Here's how the part is built. I have some questions about the finished solid (model axes, mm). Face numbers are marked on the shaded views. A direction names the side the tool comes from. Give positions to 0.01 mm unless a question says otherwise; leave off trailing zeros. Write each loop counter-clockwise with the first axis right and the second up, starting at its lowest first coordinate (ties: lowest second). Pieces come first, ordered by that corner, then holes. Notation, with made-up numbers: (87.25, 45) -> (113.25, 45) arc R22 cw to (113.25, 55) -> close; hole circle Ø9 at (88, 61). An arc over 180 degrees is marked (long way). Use one line per item in the form item = value.
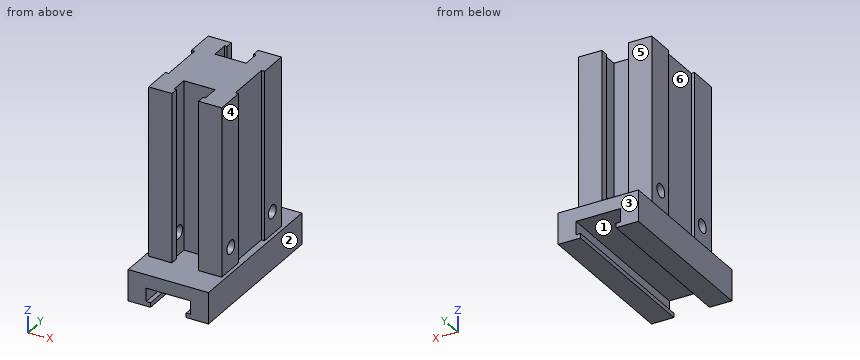
Autodesk Inventor part; units mm, degrees
ref_plane "XY Plane" through (0, 0, 0) normal (0, 0, 1) x (1, 0, 0)
sketch "Sketch1" plane through (0, 0, 0) normal (0, 0, 1) x (1, 0, 0)
  line L0 (8.2, -11.5) -> (-8.2, -11.5)
  line L1 (-8.2, -11.5) -> (-8.2, 11.5)
  line L2 (-8.2, 11.5) -> (8.2, 11.5)
  line L3 (8.2, 11.5) -> (8.2, -11.5)
  line L4 (8.2, -11.5) -> (-8.2, 11.5) construction
  line L5 (-8.2, -11.5) -> (8.2, 11.5) construction
  line L6 (8.2, -5) -> (-8.2, -5)
  line L7 (-8.2, -5) -> (-8.2, 5)
  line L8 (-8.2, 5) -> (8.2, 5)
  line L9 (8.2, 5) -> (8.2, -5)
  line L10 (8.2, -5) -> (-8.2, 5) construction
  line L11 (-8.2, -5) -> (8.2, 5) construction
  line L12 (7.5, -5) -> (-7.5, -5)
  line L13 (-7.5, -5) -> (-7.5, 5)
  line L14 (-7.5, 5) -> (7.5, 5)
  line L15 (7.5, 5) -> (7.5, -5)
  line L16 (7.5, -5) -> (-7.5, 5) construction
  line L17 (-7.5, -5) -> (7.5, 5) construction
  line L18 (3, -11.5) -> (-3, -11.5)
  line L19 (-3, -11.5) -> (-3, 11.5)
  line L20 (-3, 11.5) -> (3, 11.5)
  line L21 (3, 11.5) -> (3, -11.5)
  line L22 (3, -11.5) -> (-3, 11.5) construction
  line L23 (-3, -11.5) -> (3, 11.5) construction
  line L24 (3.5, -9.75) -> (-3.5, -9.75)
  line L25 (-3.5, -9.75) -> (-3.5, 9.75)
  line L26 (-3.5, 9.75) -> (3.5, 9.75)
  line L27 (3.5, 9.75) -> (3.5, -9.75)
  line L28 (3.5, -9.75) -> (-3.5, 9.75) construction
  line L29 (-3.5, -9.75) -> (3.5, 9.75) construction
  line L30 (3.5, -6) -> (-3.5, -6)
  line L31 (-3.5, -6) -> (-3.5, 6)
  line L32 (-3.5, 6) -> (3.5, 6)
  line L33 (3.5, 6) -> (3.5, -6)
  line L34 (3.5, -6) -> (-3.5, 6) construction
  line L35 (-3.5, -6) -> (3.5, 6) construction
  point P0 (0, 0)
  point P1 (-3, -9.75)
  point P2 (3, -9.75)
  point P3 (3, 9.75)
  point P4 (-3, 9.75)
  dimension "d0" = 23
  dimension "d1" = 16.4
  dimension "d2" = 10
  dimension "d3" = 15
  dimension "d4" = 6
  dimension "d5" = 19.5
  dimension "d6" = 7
  dimension "d7" = 12
extrude "Extrusion1" add sketch "Sketch1" along normal blind 37.8 contours L0 L21 L24 L27 L6 L3 | L0 L1 L6 L25 L24 L19 | L8 L27 L26 L21 L2 L3 | L6 L27 L8 L15 | L30 L19 L6 L21 | L21 L6 L27 L30 | L6 L21 L8 L27 | L30 L25 L6 L19 | L6 L19 L8 L21 | L8 L21 L32 L27 | L1 L2 L19 L26 L25 L8 | L13 L8 L25 L6 | L6 L25 L8 L19 | L8 L19 L32 L21 | L8 L25 L32 L19
sketch "Sketch2" plane through (0, 0, 0) normal (1, 0, 0) x (0, 1, 0)
  circle A0 centre (-8, 5) radius 1.5
  circle A1 centre (8, 5) radius 1.5
  line L0 (-6, 0) -> (-6, 37.8)
  line L1 (6, 10) -> (-6, 10)
  line L2 (-6, 10) -> (-6, 0)
  line L3 (-6, 0) -> (6, 0)
  line L4 (6, 0) -> (6, 10)
  line L5 (6, 10) -> (-6, 0) construction
  line L6 (-6, 10) -> (6, 0) construction
  point P0 (0, 0)
  point P1 (0, 5)
  point P2 (-6, 10)
  dimension "d10" = 3
  dimension "d11" = 3
  dimension "d12" = 16
  dimension "d13" = 8
  dimension "d14" = 5
  dimension "d17" = 10
extrude "Extrusion2" cut sketch "Sketch2" along normal through all both and the other way through all contours A0 | A1
sketch "Sketch3" plane through (0, 0, 0) normal (0, 0, -1) x (-1, 0, 0)
  line L0 (5, 18) -> (-5, 18)
  line L1 (-5, 18) -> (-5, -18)
  line L2 (-5, -18) -> (5, -18)
  line L3 (5, -18) -> (5, 18)
  line L4 (5, 18) -> (-5, -18) construction
  line L5 (-5, 18) -> (5, -18) construction
  line L6 (9, 18) -> (-9, 18)
  line L7 (-9, 18) -> (-9, -18)
  line L8 (-9, -18) -> (9, -18)
  line L9 (9, -18) -> (9, 18)
  line L10 (9, 18) -> (-9, -18) construction
  line L11 (-9, 18) -> (9, -18) construction
  line L12 (4, 18) -> (-4, 18)
  line L13 (-4, 18) -> (-4, -18)
  line L14 (-4, -18) -> (4, -18)
  line L15 (4, -18) -> (4, 18)
  line L16 (4, 18) -> (-4, -18) construction
  line L17 (-4, 18) -> (4, -18) construction
  point P0 (0, 0)
  point P1 (0, 18)
  point P2 (-5, 18)
  dimension "d20" = 10
  dimension "d21" = 18
  dimension "d22" = 36
  dimension "d23" = 36
  dimension "d24" = 8
extrude "Extrusion4" add sketch "Sketch3" along normal blind 7 contours L3 L2 L15 L0 | L6 L9 L8 L3 | L13 L2 L1 L0 | L1 L8 L7 L6
extrude "Extrusion5" cut sketch "Sketch3" along normal blind 6 contours L3 L2 L15 L0 | L13 L2 L1 L0
extrude "Extrusion6" add sketch "Sketch3" along normal blind 3 contours L3 L2 L15 L0 | L15 L2 L13 L0 | L13 L2 L1 L0
properties part number "Cylinder" material "Aluminum 6061"
Q1. I want a section at C-C, the plane x = -1.75. Write out the boundary of the cut face in (y, z), and give its area (3 significant figures).
Result set:
outline = (-18, -3) -> (18, -3) -> (18, 0) -> (6, 0) -> (6, 37.8) -> (-6, 37.8) -> (-6, 0) -> (-18, 0) -> close
area = 562 mm2
Q2. Will these pins go through, and if not, where does the flat tip stop? pin 1 Ø4 at (x, z) = (-5.5, 11) entering from +Y; pin 2 Ø4 at (y, z) = (8.5, 11) entering from -X; pin 3 Ø8 at (y, z) = (14, 28) entering from +X; pin 4 Ø2.5 at (y, z) = (8, 5) entering from +X.
Result set:
pin_1 = 11.5
pin_2 = -8.2
pin_3 = 8.2
pin_4 = through
Q3. Which directions (+Z, -Z, +X, -X, +Y, -Y) give clear straight access to the entire face, cutting with the end or side of a thin tool? Please do the marked faces 4, 5 and 6.
Result set:
face_4 = +Z, +X, +Y, -Y
face_5 = +Z, +X, -X, +Y
face_6 = +Z, -X
Q4. If we mould it in two halves opening along X, with no side actions, what happens to the marked faces 1, 2 and 3? For each: +X half, -X half, draft (parallel to the pull), parting line (faces both ways), or undercut.
Result set:
face_1 = undercut
face_2 = +X half
face_3 = draft
Q5. I want a section at D-D, the plane z = 12.5. Write out the boundary of the cut face in (x, y), and give its area (3 significant figures).
Result set:
outline = (-8.2, -11.5) -> (-3, -11.5) -> (-3, -9.75) -> (-3.5, -9.75) -> (-3.5, -6) -> (3.5, -6) -> (3.5, -9.75) -> (3, -9.75) -> (3, -11.5) -> (8.2, -11.5) -> (8.2, -5) -> (7.5, -5) -> (7.5, 5) -> (8.2, 5) -> (8.2, 11.5) -> (3, 11.5) -> (3, 9.75) -> (3.5, 9.75) -> (3.5, 6) -> (-3.5, 6) -> (-3.5, 9.75) -> (-3, 9.75) -> (-3, 11.5) -> (-8.2, 11.5) -> (-8.2, 5) -> (-7.5, 5) -> (-7.5, -5) -> (-8.2, -5) -> close
area = 290 mm2
Q6. I want a section at A-A, the plane x = 5.5. Write out the boundary of the cut face in (y, z), and give its area (3 significant figures).
Result set:
outline = (-18, -7) -> (18, -7) -> (18, 0) -> (11.5, 0) -> (11.5, 37.8) -> (-11.5, 37.8) -> (-11.5, 0) -> (-18, 0) -> close; hole circle Ø3 at (-8, 5); hole circle Ø3 at (8, 5)
area = 1,110 mm2
Q7. If I drill on line 1 along Y through (x, z) = (7.3, 5); line 2 along Z through (x, y) = (4.6, 8); line 3 along Z through (x, y) = (-6, -8), over which ranges is the centre line in solid material (lowest first)? Write a range as from..to.
Result set:
line_1 = -11.5..-9.5, -6.5..6.5, 9.5..11.5
line_2 = -7..-6, -3..3.5, 6.5..37.8
line_3 = -7..3.5, 6.5..37.8
Q8. I want a section at B-B, the plane y = -8. Write out the boundary of the cut face in (x, z).
Result set:
outline = (-9, -7) -> (-4, -7) -> (-4, -6) -> (-5, -6) -> (-5, -3) -> (5, -3) -> (5, -6) -> (4, -6) -> (4, -7) -> (9, -7) -> (9, 0) -> (8.2, 0) -> (8.2, 3.5) -> (3.5, 3.5) -> (3.5, 0) -> (-3.5, 0) -> (-3.5, 3.5) -> (-8.2, 3.5) -> (-8.2, 0) -> (-9, 0) -> close; (-8.2, 6.5) -> (-3.5, 6.5) -> (-3.5, 37.8) -> (-8.2, 37.8) -> close; (3.5, 6.5) -> (8.2, 6.5) -> (8.2, 37.8) -> (3.5, 37.8) -> close
